Here's how the part is built. I have some questions about the finished solid (model axes, mm). Face numbers are marked on the shaded views. A direction names the side the tool comes from. Give positions to 0.01 mm unless a question says otherwise; leave off trailing zeros. Write each loop counter-clockwise with the first axis right and the second up, starting at its lowest first coordinate (ties: lowest second). Pieces come first, ordered by that corner, then holes. Notation, with made-up numbers: (58.5, 21) -> (102.5, 21) arc R21 ccw to (102.5, 36) -> close; hole circle Ø4 at (-26.75, 82). An arc over 180 degrees is marked (long way). Answer as CSV lines item,"result". Start each with the question number.
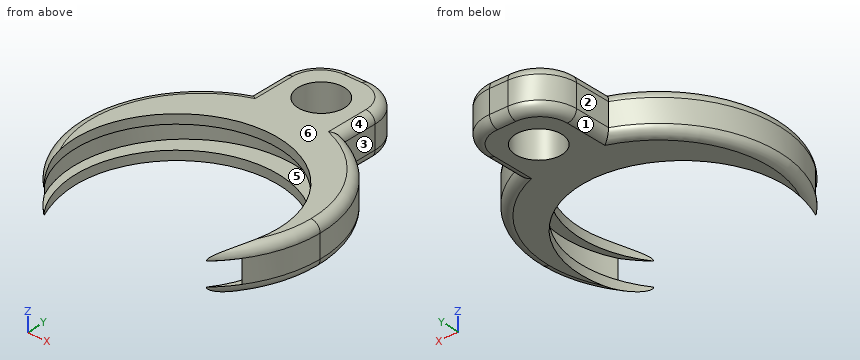
from build123d import *

# Parameters (mm, degrees)
F1_DEPTH  = 4.5
F2_R      = 4
F3_R      = 2.5
F4_DEPTH  = 4.501
F5_R      = 11
F6_DEPTH  = 1
F7_R      = 12
F8_DEPTH  = 2.5
F9_R      = 11
F10_DEPTH = 1.001
F11_R     = 0.99999


# Not quite as in the source:
# - a fillet or chamfer is up to 0.001 mm smaller than in the source, because OpenCascade refuses the exact size


with BuildPart() as f1:
    # F0 (on Top) → F1 (new body)
    with BuildSketch(Plane.XY):
        with BuildLine():
            ThreePointArc((-5, 12), (-7.2111025509, -10.8166538264), (13, 0))
            ThreePointArc((13, 0), (10.8166538264, 7.2111025509), (5, 12))
            Line((5, 12), (-5, 12))
        make_face()
        with BuildLine():
            Line((-5, 12), (5, 12))
            ThreePointArc((5, 12), (0, 13), (-5, 12))
        make_face()
        with BuildLine():
            ThreePointArc((-5, 12), (0, 13), (5, 12))
            Line((5, 12), (5, 20))
            Line((5, 20), (-5, 20))
            Line((-5, 20), (-5, 12))
        make_face()
    extrude(amount=F1_DEPTH)

    # F2
    f2_edges = [f1.edges().sort_by_distance(p)[0] for p in [
        (5, 20, 2.25),
        (-5, 20, 2.25),
    ]]
    fillet(f2_edges, radius=F2_R)

    # F3 (on face) → F4 (cut, through all)
    with BuildSketch(Plane.XY.offset(4.5)):
        with Locations((0, 15)):
            Circle(F3_R)
    extrude(amount=-F4_DEPTH, mode=Mode.SUBTRACT)

    # F5 (on face) → F6 (cut)
    with BuildSketch(Plane.XY.offset(4.5)):
        with Locations((0, -3)):
            Circle(F5_R)
    extrude(amount=-F6_DEPTH, mode=Mode.SUBTRACT)

    # F7 (on face) → F8 (cut)
    with BuildSketch(Plane.XY.offset(3.5)):
        with Locations((0, -2)):
            Circle(F7_R)
    extrude(amount=-F8_DEPTH, mode=Mode.SUBTRACT)

    # F9 (on face) → F10 (cut, through all)
    with BuildSketch(Plane.XY.offset(1)):
        with Locations((0, -3)):
            Circle(F9_R)
    extrude(amount=-F10_DEPTH, mode=Mode.SUBTRACT)

    # F11 (radius 1 in the source; OpenCascade refuses exactly that, so slightly less here)
    f11_edges = [f1.edges().sort_by_distance(p)[0] for p in [
        (12.793956, 2.305363, 4.5),
        (5, 14, 4.5),
        (-12.793956, 2.305363, 4.5),
        (12.793956, 2.305363, 0),
        (-12.793956, 2.305363, 0),
        (-3.828427, 18.828427, 0),
    ]]
    fillet(f11_edges, radius=F11_R)


solid = f1.part
Item 1: If we section it at A-A (x = 0): Please give me the cut outline in (y, z).
Item 2: If we section it at C-C (z = 1.4): Please give me the cut outline in (x, y).
Item 3: For the marked faces 1, 2 and 3, which set-ups out of +Z, -Z, +X, -X, +Y, -Y let a thin tool reach every point of the face, with its end or its side?
Item 4: If I drill on line 1 (Z direction, x = -10, y = 4.25); line 2 (Y direction, x = 0, z = 2.25); line 3 (X direction, y = -3, z = 0.75), over which ranges is the centre line in solid material (lowest first)? Write a range as [from, to].
Item 5: If we section it at B-B (y = 15): Please give me the cut outline in (x, z), and give its area (3 significant figures).
Item 6: We'd pull the mould along X, two halves only. Please class the marked faces 4, 5 and 6: released by +X, released by -X, zero draft, split by the parting line, or undercut.
Item 7: I'm going to push flat-ended pins straight in: pin 1 (15.5 mm diameter, centred on x = -0.5, y = -4, fed in from +Z); pin 2 (2 mm diameter, centred on y = 14, z = 2, fed in from -X); pin 3 (1.5 mm diameter, centred on x = 1, z = 2, fed in from -Y); pin 4 (1.5 mm diameter, centred on x = -10, z = 2.5, fed in from +Y). Where does each tip first touch, or does it pass through?
Final values:
1,outline,"(8, 0) -> (12.5, 0) -> (12.5, 4.5) -> (8, 4.5) -> (8, 3.5) -> (10, 3.5) -> (10, 1) -> (8, 1) -> close; (17.5, 0) -> (19, 0) arc R1 ccw to (20, 1) -> (20, 3.5) arc R1 ccw to (19, 4.5) -> (17.5, 4.5) -> close"
2,outline,"(-10.79, -7.25) arc R12 cw (long way) to (10.79, -7.25) arc R13 ccw to (5, 12) -> (5, 16) arc R4 ccw to (1, 20) -> (-1, 20) arc R4 ccw to (-5, 16) -> (-5, 12) arc R13 ccw to start; hole circle Ø5 at (0, 15)"
3,face 1,"-Z, -X, +Y"
3,face 2,"+Z, -Z, -X, +Y"
3,face 3,"+Z, -Z, +X, +Y"
4,line 1,"[0, 1], [3.5, 4.5]"
4,line 2,"[10, 12.5], [17.5, 20]"
4,line 3,"[-12.62, -11], [11, 12.62]"
5,outline,"(-5, 1) arc R1 ccw to (-4, 0) -> (-2.5, 0) -> (-2.5, 4.5) -> (-4, 4.5) arc R1 ccw to (-5, 3.5) -> close; (2.5, 0) -> (4, 0) arc R1 ccw to (5, 1) -> (5, 3.5) arc R1 ccw to (4, 4.5) -> (2.5, 4.5) -> close"
5,area,"21.6 mm2"
6,face 4,"released by +X"
6,face 5,"undercut"
6,face 6,"zero draft"
7,pin 1,"through"
7,pin 2,"x = -5"
7,pin 3,"y = 9.87"
7,pin 4,"y = 9.13"
